Autodesk Fusion 360 part; units mm, degrees
sketch "Sketch1" plane through (0, 0, 0) normal (0, 1, 0) x (1, 0, 0)
  line L0 (0, 0) -> (25.4, 0)
  line L1 (25.4, 0) -> (25.4, -25.4)
  line L2 (25.4, -25.4) -> (0, -25.4)
  line L3 (0, -25.4) -> (0, 0)
  dimension "d1" = 25.4
  dimension "d2" = 25.4
extrude "Extrude1" add sketch "Sketch1" along normal blind 10 makes body 1
sketch "Sketch2" plane through (0, 10, 0) normal (0, 1, 0) x (-1, 0, 0)
  line L0 (0, 25.4) -> (-25.4, 25.4)
  line L1 (-25.4, 25.4) -> (-25.4, 0)
  line L2 (-25.4, 0) -> (0, 0)
  line L3 (0, 0) -> (0, 25.4)
sketch "Sketch3" plane through (0, 0, 0) normal (-1, 0, 0) x (0, 0, 1)
  line L0 (0, 0) -> (25.4, 0)
  line L1 (25.4, 0) -> (25.4, 10)
  line L2 (25.4, 10) -> (0, 10)
  line L3 (0, 10) -> (0, 0)
  line L4 (0, 10) -> (25.4, 10)
  line L5 (25.4, 10) -> (25.4, 8.25)
  line L6 (25.4, 8.25) -> (0, 8.25)
  line L7 (0, 8.25) -> (0, 10)
  line L8 (0, 0) -> (25.4, 0)
  line L9 (25.4, 0) -> (25.4, 1.75)
  line L10 (25.4, 1.75) -> (0, 1.75)
  line L11 (0, 1.75) -> (0, 0)
  dimension "d5" = 1.75
  dimension "d6" = 1.75
extrude "Extrude2" cut sketch "Sketch3" against normal blind 6.35 contours L1 L3 L6 L10 bodies 1
sketch "Sketch4" plane through (25.4, 0, 0) normal (1, 0, 0) x (0, 0, -1)
  line L0 (-25.4, 0) -> (0, 0)
  line L1 (0, 0) -> (0, 10)
  line L2 (0, 10) -> (-25.4, 10)
  line L3 (-25.4, 10) -> (-25.4, 0)
  line L4 (-25.4, 10) -> (0, 10)
  line L5 (0, 10) -> (0, 8.25)
  line L6 (0, 8.25) -> (-25.4, 8.25)
  line L7 (-25.4, 8.25) -> (-25.4, 10)
  line L8 (-25.4, 0) -> (0, 0)
  line L9 (0, 0) -> (0, 1.75)
  line L10 (0, 1.75) -> (-25.4, 1.75)
  line L11 (-25.4, 1.75) -> (-25.4, 0)
  dimension "d9" = 1.75
  dimension "d10" = 25.4
  dimension "d11" = 1.75
extrude "Extrude3" cut sketch "Sketch4" against normal blind 6.35 contours L1 L3 L6 L10 bodies 1
copy_body "Body->Comp1" bodies 1 removing the originals makes body 2 in component "Half inch spacer"
component "Half inch spacer" placed x (1, 0, 0) y (0, 1, 0) z (0, 0, 1) at (0, 0, 0)
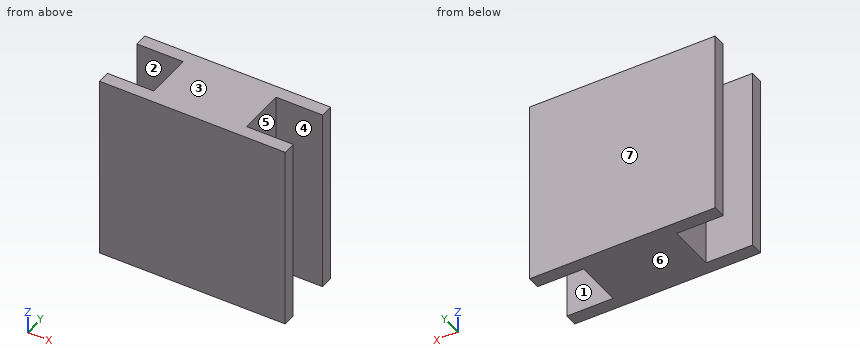
Verification items for the finished model (mm, model axes). Face numbers are marked on the shaded views. A direction names the side the tool comes from. Coordinates: 2 decimals unless noted, no trailing zeros. Order: outer loops, then holes, each group sorted by start corner. A loop starts at its lowest first (then second) coordinate and runs counter-clockwise, first axis right, second up. Notation, with made-up numbers: (-25.5, 82) - (22.5, 82) arc R20 ccw to (22.5, 113) - close; hole circle Ø6 at (-27, -33.75). An arc over 180 degrees is marked (long way). Return JSON: item names as keys, results as strings.
(1) Section check C-C, the plane y = 3.25. Record the cut outline in (x, z), and give its area (3 significant figures).
Filled sheet:
{"outline": "(6.35, 0) - (19.05, 0) - (19.05, 25.4) - (6.35, 25.4) - close", "area": "323 mm^2"}
(2) Section check B-B, the plane z = 5.5. Record the cut outline in (x, y).
Filled sheet:
{"outline": "(0, 0) - (25.4, 0) - (25.4, 1.75) - (19.05, 1.75) - (19.05, 8.25) - (25.4, 8.25) - (25.4, 10) - (0, 10) - (0, 8.25) - (6.35, 8.25) - (6.35, 1.75) - (0, 1.75) - close"}
(3) Mould release check, pull along Y, two halves, no side actions. Record for the marked faces 4, 5, 6 and 7: pulls with the +Y half, pulls with the -Y half, needs draft (parallel to the pull), parting line crosses it, or undercut.
Filled sheet:
{"face 4": "undercut", "face 5": "undercut", "face 6": "needs draft", "face 7": "pulls with the +Y half"}
(4) Access from +Z, -Z, +X, -X, +Y, -Y to the whole of each face (thin tool, end or side, straight path). Record for the marked faces 1, 2 and 3.
Filled sheet:
{"face 1": "+Z, -Z, +X", "face 2": "+Z, -Z, -X", "face 3": "+Z, +X, -X, +Y, -Y"}
(5) Go/stop test with flat-tipped pins: pin 1 (2 mm diameter, centred on y = 5, z = 12.5, fed in from -X); pin 2 (2 mm diameter, centred on y = 3.5, z = 18.5, fed in from +X). Record where each tip stops, or that it passes through.
Filled sheet:
{"pin 1": "stops at x = 6.35", "pin 2": "stops at x = 19.05"}
(6) Section check A-A, the plane x = 20.75. Record the cut outline in (y, z).
Filled sheet:
{"outline": "(0, 0) - (1.75, 0) - (1.75, 25.4) - (0, 25.4) - close; (8.25, 0) - (10, 0) - (10, 25.4) - (8.25, 25.4) - close"}
(7) Thickness scan on line 1 along Y through (x, z) = (21.5, 6.25); line 2 along X through (y, z) = (6.5, 7.5). Record the ranges inside material, lowest first.
Filled sheet:
{"line 1": "y = 0 to 1.75, 8.25 to 10", "line 2": "x = 6.35 to 19.05"}
